```python
from build123d import *

# Parameters (mm, degrees)
SKETCH_1_R      = 1.6
EXTRUDE_1_DEPTH = 1.5


with BuildPart() as part:
    # Эскиз1 → Бобышка-Вытянуть1 (new body)
    with BuildSketch(Plane.XY):
        with BuildLine():
            Line((0, 20.99999864), (0, 0))
            Line((0, 0), (79, 0))
            Line((79, 0), (79, 25.0000008))
            Line((79, 25.0000008), (65.525211558, 25.0000008))
            ThreePointArc((65.525211558, 25.0000008), (48.741944539, 14.922513652), (29.408996509, 17.99999956))
            Line((29.408996509, 17.99999956), (20.000212839, 17.99999956))
            ThreePointArc((20.000212839, 17.99999956), (19.617529225, 18.076120064), (19.293105722, 18.292892918))
            Line((19.293105722, 18.292892918), (16.586, 20.99999864))
            Line((16.586, 20.99999864), (0, 20.99999864))
        make_face()
        with Locations((3.5, 6)):
            Circle(SKETCH_1_R, mode=Mode.SUBTRACT)
        with Locations((13, 8)):
            Circle(SKETCH_1_R, mode=Mode.SUBTRACT)
    extrude(amount=EXTRUDE_1_DEPTH)


solid = part.part
```
For this review, take the finished solid that the model builds, in its own axes (mm). A direction names the side the tool comes from. Coordinates: 2 decimals unless noted, no trailing zeros. Loops run counter-clockwise (first coordinate to the right, second up) from the corner with the lowest first, then second, coordinate; pieces in that order, holes last.
1. Insertion check: P1, Ø0.8, axis at x = 23.5, z = 1, coming from the +Y side. The pin has a flat end and moves straight along its axis. Give the tip position at first contact, or say it passes through.
2. Mouldability with a two-part tool opening along X and no side actions: class faces 4 (the flat face through (39, 0, 1)), 5 (the cylindrical face through (11.4, 8.07, 0.74)), 6 (the flat face through (0, 11, 1)) as +X half, -X half, draft (parallel to the pull), parting line (faces both ways), or undercut.
3. Add section B-B, the plane z = 0.25. Give the boundary of the cut face in (x, y), then the cut area to 3 significant figures.
4. For faces 1 (the flat face through (8, 21, 1)), 2 (the flat face through (39, 10, 0)), 3 (the flat face through (25, 18, 1)), list the 3-axis set-ups (+Z, -Z, +X, -X, +Y, -Y) from which the entire face can be reached by the end or side of a thin tool; tool diameter is ignored.
5. Add section C-C, the plane y = 17. Give the boundary of the cut face in (x, z).
6. Add section D-D, the plane x = 39. Give the boundary of the cut face in (y, z), then the cut area to 3 significant figures.
7. Add section A-A, the plane x = 13. Give the boundary of the cut face in (y, z), then the cut area to 3 significant figures.
8. For line 1 (Y direction, x = 13, z = 0.75); line 2 (X direction, y = 19, z = 0.8); line 3 (X direction, y = 17.5, z = 0.9), list the stretches that pass through material, from the lowest coordinate up.
Result:
1. P1: stops at y = 18
2. face 4: draft
2. face 5: undercut
2. face 6: -X half
3. outline: (0, 0) - (79, 0) - (79, 25) - (65.53, 25) arc R28.6 cw to (29.41, 18) - (20, 18) arc R1 cw to (19.29, 18.29) - (16.59, 21) - (0, 21) - close; hole circle Ø3.2 at (3.5, 6); hole circle Ø3.2 at (13, 8)
3. area: 1,510 mm2
4. face 1: +Z, -Z, -X, +Y
4. face 2: -Z, +X, -X, +Y, -Y
4. face 3: +Z, -Z, +Y
5. outline: (0, 0) - (31.39, 0) - (31.39, 1.5) - (0, 1.5) - close; (55.21, 0) - (79, 0) - (79, 1.5) - (55.21, 1.5) - close
6. outline: (0, 0) - (14.73, 0) - (14.73, 1.5) - (0, 1.5) - close
6. area: 22.1 mm2
7. outline: (0, 0) - (6.4, 0) - (6.4, 1.5) - (0, 1.5) - close; (9.6, 0) - (21, 0) - (21, 1.5) - (9.6, 1.5) - close
7. area: 26.7 mm2
8. line 1: y = 0 to 6.4, 9.6 to 21
8. line 2: x = 0 to 18.59, 58.86 to 79
8. line 3: x = 0 to 30.35, 56.25 to 79
